Autodesk Inventor part; units mm, degrees
ref_plane "YZ-Ebene" through (0, 0, 0) normal (1, 0, 0) x (0, 1, 0)
ref_plane "XZ-Ebene" through (0, 0, 0) normal (0, 1, 0) x (-1, 0, 0)
ref_plane "XY-Ebene" through (0, 0, 0) normal (0, 0, 1) x (1, 0, 0)
sketch "Skizze1" plane through (0, 0, 0) normal (0, 0, 1) x (1, 0, 0)
  line L0 (-4.8497, 0) -> (4.8497, 0)
  line L1 (0, -5.6) -> (0, 5.6)
  line L2 (0, 4) -> (3.4641, 2)
  line L3 (3.4641, 2) -> (3.4641, -2)
  line L4 (3.4641, -2) -> (0, -4)
  line L5 (0, -4) -> (-3.4641, -2)
  line L6 (-3.4641, -2) -> (-3.4641, 2)
  line L7 (-3.4641, 2) -> (0, 4)
  point P0 (0, 0)
  dimension "d9" = 8
extrude "Extrusion1" add sketch "Skizze1" along normal blind 3.5
sketch "Skizze2" plane through (0, 0, 3.5) normal (0, 0, 1) x (1, 0, 0)
  line L0 (3.4641, 2) -> (0, 4)
  circle A0 centre (0, 0) radius 3.4641
extrude "Extrusion2" cut sketch "Skizze2" against normal blind 3.5 draft 45 keep common part
sketch "Skizze3" plane through (0, 0, 0) normal (0, 0, -1) x (-1, 0, 0)
  circle A0 centre (0, 0) radius 2.5
  dimension "d6" = 5
extrude "Extrusion3" add sketch "Skizze3" along normal blind 20
chamfer "Fase1" distance 0.5 angle 45 1 edges at (2.5, 0, -20)
thread "Gewinde1"
thread "Gewinde2"
thread "Gewinde3"
properties part number "Sechskantenschraube_ra8846s" material "Stahl, hochfest, niedrig legiert"
CAD build for the part. Positions are in the model's coordinates, mm. A direction names the side the tool comes from. Round coordinates to 2 decimals unless told otherwise and drop trailing zeros. Order: outer loops, then holes, each group sorted by start corner. A loop starts at its lowest first (then second) coordinate and runs counter-clockwise, first axis right, second up. Notation, with made-up numbers: (65.25, -25.75) - (105.25, -25.75) arc R16 ccw to (105.25, -12.75) - close; hole circle Ø3 at (-36, -24.5). An arc over 180 degrees is marked (long way). Answer as CSV lines item,"result". Start each with the question number.
1. Drill centre lines: L1, parallel to Y at x = 1.5, z = -9.5; L2, parallel to Z at x = -2.5, y = 1.25. Where is each one in solid material? Low to high. Write a range as [from, to].
2. Tool access for faces 1 (the face through (0, -3, 0)), 2 (the face through (-0.009, 3.594, 3.37)): list every direction of +Z, -Z, +X, -X, +Y, -Y with a clear straight run to the whole face (end or side of a thin tool).
3. Saw through at A-A, the plane z = -0.5. Write the cut outline in (x, y), and give its area (3 significant figures).
4. Pin check, flat tips, straight feed: pin 1 (1 mm diameter, centred on x = -2.5, z = -9.5, fed in from -Y); pin 2 (1.5 mm diameter, centred on x = 2.5, z = -7, fed in from -Y); pin 3 (1 mm diameter, centred on y = -2.5, z = -11, fed in from -X). Stop position of each tip, or through.
Model answer:
1,L1,"y = [-2, 2]"
1,L2,"z = [0, 3.5]"
2,face 1,"-Z"
2,face 2,"+Z, +Y"
3,outline,"circle Ø5 at (0, 0)"
3,area,"19.6 mm²"
4,pin 1,"stops at y = -1.5"
4,pin 2,"stops at y = -1.79"
4,pin 3,"stops at x = -1.5"
